Input: part model. Units: mm. Frame: model coordinates. A direction names the side the tool comes from. Round coordinates to 2 decimals unless told otherwise and drop trailing zeros. Loops run counter-clockwise (first coordinate to the right, second up) from the corner with the lowest first, then second, coordinate; pieces in that order, holes last. Notation, with made-up numbers: M 11,73.5 L 29,73.5 A8 cw 29,83.5 Z; hole C -21.75,1.5 d8. An arc over 180 degrees is marked long. Put each result on its own line as item: value. Start each with the question number.
1) Reachability of faces 5 (the face through (40.73, 6.26, -62.61)), 6 (the face through (45, 18, -76.2)), 7 (the face through (9.39, 79.37, -101.32)), 8 (the face through (16, 41, -76.2)) from +Z, -Z, +X, -X, +Y, -Y: full face, straight path, thin tool, end or side. Return the list, or none.
2) Section C-C on y = 69. Output: boundary loops of the cut face in (x, z).
3) Section D-D on z = -80.5. Output: boundary loops of the cut face in (x, y) (3 decimals), plus the area to 3 significant figures.
4) Section B-B on z = -19.05. Output: boundary loops of the cut face in (x, y).
5) Line query: probe 1 along X at (y, z) = (15.25, -50.8); probe 2 along Z at (x, y) = (31, 15); probe 3 along X at (y, z) = (59.5, -83). Output: solid intervals per line, ascending.
6) Pin query (flat end, axial travel): pin 1 (5 mm diameter, centred on x = 37, z = -73.5, fed in from +Y); pin 2 (7.5 mm diameter, centred on x = 31.75, z = -50.8, fed in from -Y); pin 3 (5.5 mm diameter, centred on x = 11, y = 53, fed in from +Z); pin 4 (12 mm diameter, centred on x = 5.5, z = -24, fed in from +Y). Return the tip coordinate at first contact, or that it passes through.
7) Draft query along X for faces 1 (the face through (19.05, 58, -118)), 2 (the face through (32, 12.7, -63)), 3 (the face through (31, 19.05, -39)), 4 (the face through (22.665, 6.439, -62.611)). Return one class per face: +X half, -X half, draft (parallel to the pull), parting line (faces both ways), or undercut.
8) Section A-A on x = 20.5. Output: boundary loops of the cut face in (y, z), plus the area to 3 significant figures.
from build123d import *

# Parameters (mm, degrees)
BOSS_EXTRUDE1_DEPTH = 12.7
BOSS_EXTRUDE2_DEPTH = 50.8
BOSS_EXTRUDE3_START = 12.7
BOSS_EXTRUDE3_DEPTH = 6.35
CUT_EXTRUDE1_DEPTH  = 165.886159592
SKETCH4_R           = 6.35
CUT_EXTRUDE2_DEPTH  = 156.055766178
CUT_EXTRUDE3_DEPTH  = 50.8


# Read off the part's stored shape, not the designer's step: Boss-Extrude3
with BuildPart() as part:
    # Sketch1 → Boss-Extrude1 (new body)
    with BuildSketch(Plane(origin=(0, 0, 0), x_dir=(0, 0, -1), z_dir=(1, 0, 0))):
        with BuildLine():
            Line((0, 0), (127, 0))
            Line((127, 0), (127, 66.675))
            ThreePointArc((127, 66.675), (114.370135783, 88.631402986), (89.04065889, 88.752657278))
            Line((89.04065889, 88.752657278), (6.420329445, 41.752339853))
            ThreePointArc((6.420329445, 41.752339853), (1.721798507, 37.098579105), (0, 30.713511214))
            Line((0, 30.713511214), (0, 0))
        make_face()
        with BuildLine():
            Line((88.9, 41.275), (88.9, 66.675))
            ThreePointArc((88.9, 66.675), (101.6, 79.375), (114.3, 66.675))
            Line((114.3, 66.675), (114.3, 41.275))
            ThreePointArc((114.3, 41.275), (101.6, 28.575), (88.9, 41.275))
        make_face(mode=Mode.SUBTRACT)
    extrude(amount=BOSS_EXTRUDE1_DEPTH)

    # Sketch1_3 → Boss-Extrude2 (add)
    with BuildSketch(Plane(origin=(0, 0, 0), x_dir=(0, 0, -1), z_dir=(1, 0, 0))):
        Polygon((0, 19.05), (0, 0), (127, 0), (127, 22.225), (76.2, 22.225), (76.2, 19.05), align=None)
    extrude(amount=BOSS_EXTRUDE2_DEPTH)

    # Boss-Extrude3 outline → Boss-Extrude3 (add)
    with BuildSketch(Plane(origin=(0, 0, 0), x_dir=(0, 0, -1), z_dir=(1, 0, 0)).offset(BOSS_EXTRUDE3_START)):
        with BuildLine():
            ThreePointArc((127, 66.675), (101.6, 92.075), (76.2, 66.675))
            Line((76.2, 66.675), (76.2, 22.225))
            Line((76.2, 22.225), (127, 22.225))
            Line((127, 22.225), (127, 66.675))
        make_face()
        with BuildLine():
            Line((114.3, 66.675), (114.3, 41.275))
            ThreePointArc((114.3, 41.275), (101.6, 28.575), (88.9, 41.275))
            Line((88.9, 41.275), (88.9, 66.675))
            ThreePointArc((88.9, 66.675), (101.6, 79.375), (114.3, 66.675))
        make_face(mode=Mode.SUBTRACT)
    extrude(amount=BOSS_EXTRUDE3_DEPTH)

    # Sketch3 → Cut-Extrude1 (cut, through all)
    with BuildSketch(Plane.XY):
        Polygon((-67.157348715, -180.609598473), (37.117651581, 0), (44.45, 12.7), (19.05, 12.7), (26.382348419, 0), (130.657348715, -180.609598473), (130.657348715, 236.490402714), (-67.157348715, 236.490402714), align=None)
    extrude(amount=-CUT_EXTRUDE1_DEPTH, mode=Mode.SUBTRACT)

    # Sketch4 → Cut-Extrude2 (cut, through all)
    with BuildSketch(Plane(origin=(0, 19.05, 0), x_dir=(1, 0, 0), z_dir=(0, 1, 0))):
        with Locations(Location((31.75, 19.05, 0), (0, 0, 270))):
            Circle(SKETCH4_R)
        with Locations(Location((31.75, 50.8, 0), (0, 0, 270))):
            Circle(SKETCH4_R)
    extrude(amount=-CUT_EXTRUDE2_DEPTH, mode=Mode.SUBTRACT)

    # Sketch5 → Cut-Extrude3 (cut)
    with BuildSketch(Plane(origin=(0, 0, -127), x_dir=(-1, 0, 0), z_dir=(0, 0, -1))):
        Polygon((-19.05, 22.225), (-50.8, 13.71761314), (-50.8, 22.225), align=None)
    extrude(amount=-CUT_EXTRUDE3_DEPTH, mode=Mode.SUBTRACT)


solid = part.part
Geometry results:
1. face 5: +Z, -Z
1. face 6: -Z, +X, +Y
1. face 7: +X, -X
1. face 8: +Z, +X, +Y
2. outline: M 0,-126.89 L 19.05,-126.89 L 19.05,-114.09 L 0,-114.09 Z; M 0,-89.11 L 19.05,-89.11 L 19.05,-76.31 L 12.7,-76.31 L 12.7,-54.32 L 0,-54.32 Z
3. outline: M 0,0 L 26.382,0 L 19.05,12.7 L 44.45,12.7 L 37.118,0 L 50.8,0 L 50.8,13.718 L 19.05,22.225 L 19.05,80.815 L 12.7,80.815 L 12.7,83.894 L 0,83.894 Z
3. area: 1,920 mm²
4. outline: M 0,0 L 25.4,0 L 25.4,1.7 L 19.05,12.7 L 25.4,12.7 L 25.4,19.05 L 12.7,19.05 L 12.7,48.94 L 0,48.94 Z; M 38.1,0 L 50.8,0 L 50.8,19.05 L 38.1,19.05 L 38.1,12.7 L 44.45,12.7 L 38.1,1.7 Z
5. probe 1: x = 0 to 25.4, 38.1 to 50.8
5. probe 2: z = -127 to -57.11, -44.49 to -25.36, -12.74 to 0
5. probe 3: x = 0 to 19.05
6. pin 1: stops at y = 19.05
6. pin 2: passes through
6. pin 3: stops at z = -21.36
6. pin 4: stops at y = 55.17
7. face 1: +X half
7. face 2: undercut
7. face 3: draft
7. face 4: undercut
8. outline: M 0,-127 L 10.19,-127 L 10.19,0 L 0,0 Z; M 12.7,-127 L 21.84,-127 L 21.84,-76.2 L 19.05,-76.2 L 19.05,0 L 12.7,0 Z
8. area: 2,240 mm²
